from build123d import *

# Parameters (mm, degrees)
SKETCH1_R           = 2.6
BOSS_EXTRUDE1_DEPTH = 10
SKETCH2_R           = 1.7
BOSS_EXTRUDE2_DEPTH = 10
CUT_EXTRUDE1_DEPTH  = 3.61
CUT_EXTRUDE2_DEPTH  = 7.01


with BuildPart() as part:
    # Sketch1 → Boss-Extrude1 (new body)
    with BuildSketch(Plane.XY.offset(348)):
        with BuildLine():
            ThreePointArc((295.244800935, 76.37840131), (304.167556264, 63.635386072), (316.910571501, 72.558141401))
            add(Edge.make_bspline(
                [(316.910571501, 72.558141401), (317.993077182, 78.060080938), (319.436691833, 86.419493367), (320.644104939, 97.746663028), (321.086020795, 106.446056452), (320.974468629, 115.188631518), (320.331239752, 123.834659135), (319.294204188, 132.281931409), (318.037316746, 140.511779077), (316.695476199, 148.568110679), (314.90656957, 159.124453911), (313.612933772, 167.009808068), (312.802500789, 172.25742631)],
                knots=[0, 0, 0, 0, 0.167265195, 0.252809118, 0.339604775, 0.426899602, 0.513395067, 0.598049027, 0.680668932, 0.761679683, 0.84163696, 1, 1, 1, 1], degree=3))
            ThreePointArc((312.802500789, 172.25742631), (297.74257369, 182.802500789), (287.197499211, 167.74257369))
            add(Edge.make_bspline(
                [(287.197499211, 167.74257369), (288.245214147, 162.428752521), (289.885822364, 154.498518205), (292.118297352, 143.988320878), (293.742742512, 136.235372867), (295.2339085, 128.615976653), (296.473470386, 121.13730858), (297.336811691, 113.762401768), (297.738284398, 106.419106942), (297.668798337, 99.033764721), (297.014800417, 88.987730843), (296.022440082, 81.435185794), (295.244800935, 76.37840131)],
                knots=[0, 0, 0, 0, 0.175721332, 0.26273732, 0.348606728, 0.432722922, 0.514619289, 0.594500878, 0.673506544, 0.753057452, 0.833978021, 1, 1, 1, 1], degree=3))
        make_face()
        with Locations((300, 170)):
            Circle(SKETCH1_R, mode=Mode.SUBTRACT)
        with BuildLine():
            Line((298.037273547, 149.741721474), (301.215790437, 134.288941883))
            ThreePointArc((301.215790437, 134.288941883), (302.249879541, 132.731371076), (304.075121449, 132.326575973))
            Line((304.075121449, 132.326575973), (309.533784891, 133.235441013))
            ThreePointArc((309.533784891, 133.235441013), (311.154644108, 134.244376396), (311.590714405, 136.103133481))
            Line((311.590714405, 136.103133481), (309.035810829, 151.799472168))
            ThreePointArc((309.035810829, 151.799472168), (308.002694304, 153.44538336), (306.102883834, 153.854129723))
            Line((306.102883834, 153.854129723), (300.020607078, 152.701705588))
            ThreePointArc((300.020607078, 152.701705588), (298.409129896, 151.6370167), (298.037273547, 149.741721474))
        make_face(mode=Mode.SUBTRACT)
        with BuildLine():
            Line((303.095062376, 122.802641733), (304.478179716, 107.400584875))
            ThreePointArc((304.478179716, 107.400584875), (305.271665108, 105.787912405), (306.941989082, 105.124324138))
            Line((306.941989082, 105.124324138), (311.308057506, 105.078615953))
            ThreePointArc((311.308057506, 105.078615953), (313.134691512, 105.844024349), (313.831371675, 107.697960312))
            Line((313.831371675, 107.697960312), (313.059492575, 123.830124112))
            ThreePointArc((313.059492575, 123.830124112), (312.159795141, 125.633704646), (310.221794191, 126.187338583))
            Line((310.221794191, 126.187338583), (305.244487527, 125.502939826))
            ThreePointArc((305.244487527, 125.502939826), (303.629055674, 124.583200895), (303.095062376, 122.802641733))
        make_face(mode=Mode.SUBTRACT)
        with BuildLine():
            Line((304.341810749, 95.98294616), (302.807326902, 80.41966071))
            ThreePointArc((302.807326902, 80.41966071), (303.310735667, 78.653947907), (304.884570682, 77.708323546))
            Line((304.884570682, 77.708323546), (308.061893299, 77.17917356))
            ThreePointArc((308.061893299, 77.17917356), (309.951832836, 77.629811361), (310.948319998, 79.297731989))
            Line((310.948319998, 79.297731989), (313.173535223, 95.152129395))
            ThreePointArc((313.173535223, 95.152129395), (312.633934067, 97.081184589), (310.85135927, 97.994886096))
            Line((310.85135927, 97.994886096), (306.983305274, 98.232924126))
            ThreePointArc((306.983305274, 98.232924126), (305.208657773, 97.640818137), (304.341810749, 95.98294616))
        make_face(mode=Mode.SUBTRACT)
    extrude(amount=BOSS_EXTRUDE1_DEPTH)

    # Sketch2 → Boss-Extrude2 (add)
    with BuildSketch(Plane.XY.offset(348)):
        Polygon((294.95939437, 45.965927831), (306.777087406, 43.882149699), (311.465588203, 70.47195903), (299.647895167, 72.555737162), align=None)
        with Locations((301.736481777, 49.84807753)):
            Circle(SKETCH2_R, mode=Mode.SUBTRACT)
    extrude(amount=BOSS_EXTRUDE2_DEPTH)

    # Sketch3 → Cut-Extrude1 (cut)
    with BuildSketch(Plane.XY.offset(354.4)):
        Polygon((304.734272207, 170), (302.367136104, 174.1), (297.632863896, 174.1), (295.265727793, 170), (297.632863896, 165.9), (302.367136104, 165.9), align=None)
    extrude(amount=CUT_EXTRUDE1_DEPTH, mode=Mode.SUBTRACT)

    # Sketch4 → Cut-Extrude2 (cut)
    with BuildSketch(Plane.XY.offset(351)):
        with BuildLine():
            ThreePointArc((300.580931265, 81.888864063), (306.130868326, 74.323372231), (313.696360158, 79.873309293))
            add(Edge.make_bspline(
                [(313.696360158, 79.873309293), (314.375332718, 83.768049726), (315.269853801, 89.655581864), (316.076109947, 97.581166828), (316.452007736, 103.60449348), (316.564187736, 109.663923395), (316.399741723, 115.723723037), (315.97594992, 121.744253087), (315.33821911, 127.695568385), (314.545946492, 133.565929662), (313.36456358, 141.260072259), (312.394961182, 146.988748853), (311.75464163, 150.792263987)],
                knots=[0, 0, 0, 0, 0.166088556, 0.250039022, 0.33458405, 0.419536565, 0.504540949, 0.589152475, 0.673005298, 0.755933527, 0.837970837, 1, 1, 1, 1], degree=3))
            ThreePointArc((311.75464163, 150.792263987), (302.327575287, 157.208623235), (295.911216039, 147.781556891))
            add(Edge.make_bspline(
                [(295.911216039, 147.781556891), (296.697686325, 144.058532846), (297.878134482, 138.498789725), (299.330987648, 131.099349657), (300.305049322, 125.614550146), (301.11991691, 120.165560812), (301.730137241, 114.739277873), (302.103500244, 109.317606169), (302.228444831, 103.882909759), (302.114203921, 98.423103229), (301.672760974, 91.075496307), (301.065579784, 85.565175403), (300.580931265, 81.888864063)],
                knots=[0, 0, 0, 0, 0.171659874, 0.256391336, 0.340162967, 0.422938325, 0.504894902, 0.58642712, 0.668013916, 0.750042635, 0.832709798, 1, 1, 1, 1], degree=3))
        make_face()
    extrude(amount=CUT_EXTRUDE2_DEPTH, mode=Mode.SUBTRACT)


solid = part.part
Geometry check sheet. Reference: the model listing, model coordinates, mm. A direction names the side the tool comes from. Give positions to 0.01 mm unless a question says otherwise; leave off trailing zeros. Use one line per item in the form item = value.
1) Access from +Z, -Z, +X, -X, +Y, -Y to the whole of each face (thin tool, end or side, straight path). Record for faces 1 (the face through (300.786, 44.939, 352.93)), 2 (the face through (311.139, 134.222, 349.479)), 3 (the face through (300, 165.9, 356)).
Working result:
face_1 = +Z, -Z, -X, -Y
face_2 = +Z, -Z
face_3 = +Z
2) Depth check by flat-ended pin: pin 1 Ø6 at (y, z) = (140, 356.5) entering from -X; pin 2 Ø4 at (x, z) = (301, 356.5) entering from -Y; pin 3 Ø4 at (y, z) = (152, 351) entering from -X. Enter the tip coordinate at first touch or a pass-through.
Working result:
pin_1 = 292.32
pin_2 = 44.55
pin_3 = 290
3) Sectioned sample at A-A (z = 356.25). Count the separate pieces of the cut face and the enclosed holes in it, and give its area (3 significant figures).
Working result:
separate_pieces = 1
enclosed_holes = 3
area = 1,750 mm^2
4) Draft check along Y on faces 4 (the face through (300, 174.1, 356)), 5 (the face through (308.025, 153.429, 349.479)), 6 (the face through (308.556, 53.971, 352.93)). Enter one of: released by +Y, released by -Y, zero draft, split by the parting line, or undercut.
Working result:
face_4 = undercut
face_5 = undercut
face_6 = released by -Y
5) Material ranges on probe 1 along X at (y, z) = (170, 349.5); probe 2 along Y at (x, z) = (303, 357.5); probe 3 along X at (y, z) = (131.5, 353.25), recorded low to high. Write a range as from..to.
Working result:
probe_1 = 287..297.4, 302.6..313.15
probe_2 = 44.55..48.71, 50.99..75.7, 157.31..167, 173..182.65
probe_3 = 294.66..299.24, 314.82..319.36
